Geometry: final body of the model. Coordinates: model frame, mm. Face numbers are marked on the shaded views. A direction names the side the tool comes from. Give positions to 0.01 mm unless a question says otherwise; leave off trailing zeros. Loops run counter-clockwise (first coordinate to the right, second up) from the corner with the lowest first, then second, coordinate; pieces in that order, holes last.
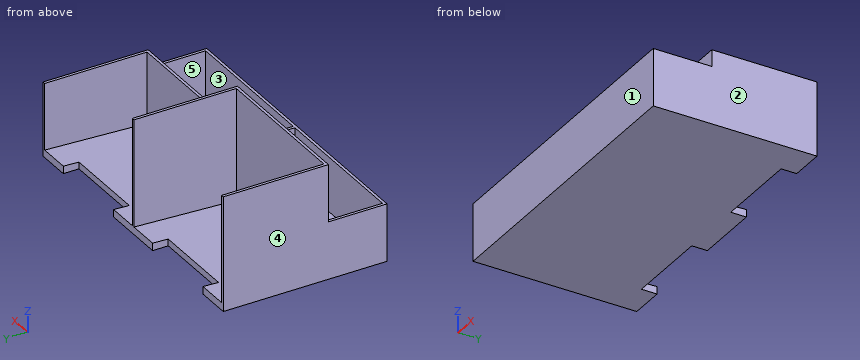
```python
from build123d import *

# Parameters (mm, degrees)
SKETCH1_W               = 193.4
SKETCH1_H               = 104.8
BOSS_EXTRUDE1_DEPTH     = 1.8
SKETCH1_8_W             = 1.8
SKETCH1_8_H             = 65.5
SKETCH1_8_H_2           = 1.8
SKETCH1_8_W_2           = 94
BOSS_EXTRUDE2_DEPTH     = 71.7
SKETCH1_10_W            = 94
SKETCH1_10_H            = 1.8
SKETCH1_10_W_2          = 1.8
SKETCH1_10_H_2          = 65.5
BOSS_EXTRUDE3_DEPTH     = 45.7
BOSS_EXTRUDE4_DEPTH     = 35
BOSS_EXTRUDE8_REACH     = 231.858
CUT_EXTRUDE1_DEPTH      = 27
CUT_EXTRUDE1_DEPTH_BACK = 16
SKETCH1_12_W            = 54
SKETCH1_12_H            = 10


with BuildPart() as part:
    # Sketch1 → Boss-Extrude1 (new body)
    with BuildSketch(Plane.XY):
        with Locations((96.7, 52.4)):
            Rectangle(SKETCH1_W, SKETCH1_H)
    extrude(amount=-BOSS_EXTRUDE1_DEPTH)

    # Sketch1<8> → Boss-Extrude2 (add)
    with BuildSketch(Plane.XY):
        with Locations((96.7, 72.05)):
            Rectangle(SKETCH1_8_W, SKETCH1_8_H)
        with Locations((96.7, 38.4)):
            Rectangle(SKETCH1_8_W, SKETCH1_8_H_2)
        with Locations((48.8, 38.4)):
            Rectangle(SKETCH1_8_W_2, SKETCH1_8_H_2)
        with Locations((0.9, 72.05)):
            Rectangle(SKETCH1_8_W, SKETCH1_8_H)
        with Locations((0.9, 38.4)):
            Rectangle(SKETCH1_8_W, SKETCH1_8_H_2)
    extrude(amount=BOSS_EXTRUDE2_DEPTH)

    # Sketch1<10> → Boss-Extrude3 (add)
    with BuildSketch(Plane.XY):
        with Locations((144.6, 38.4)):
            Rectangle(SKETCH1_10_W, SKETCH1_10_H)
        with Locations((192.5, 72.05)):
            Rectangle(SKETCH1_10_W_2, SKETCH1_10_H_2)
        with Locations((192.5, 38.4)):
            Rectangle(SKETCH1_10_W_2, SKETCH1_10_H)
    extrude(amount=BOSS_EXTRUDE3_DEPTH)

    # Sketch1<11> → Boss-Extrude4 (add)
    with BuildSketch(Plane.XY):
        Polygon((0, 37.5), (0, 0), (193.4, 0), (193.4, 37.5), (191.6, 37.5), (191.6, 1.8), (97.6, 1.8), (97.6, 37.5), (95.8, 37.5), (95.8, 1.8), (1.8, 1.8), (1.8, 37.5), align=None)
    extrude(amount=BOSS_EXTRUDE4_DEPTH)

    # Boss-Extrude8: up to this face of the body (flat: up to its plane)
    boss_extrude8_end = Plane(part.part.faces().sort_by_distance((1.8, 72.05, 35.85))[0])
    # Sketch2 → Boss-Extrude8 (add, up to the picked face)
    with BuildSketch(Plane.ZY.offset(-191.6), mode=Mode.PRIVATE) as boss_extrude8_sk1:
        Polygon((3, 104.8), (0, 104.8), (0, 39.3), align=None)
    boss_extrude8_tool1 = split(extrude(boss_extrude8_sk1.sketch, amount=BOSS_EXTRUDE8_REACH, mode=Mode.PRIVATE), bisect_by=boss_extrude8_end, keep=Keep.BOTH, mode=Mode.PRIVATE)
    add(boss_extrude8_tool1.solids().sort_by(Axis((191.6, 82.966667, 1), (-1, 0, 0)))[0])

    # Sketch1<12> → Cut-Extrude1 (cut, two sides: drawn at the far end of the back side and taken through both)
    with BuildSketch(Plane.XY.offset(-CUT_EXTRUDE1_DEPTH_BACK)):
        with Locations((144.6, 99.8)):
            Rectangle(SKETCH1_12_W, SKETCH1_12_H)
        with Locations((48.8, 99.8)):
            Rectangle(SKETCH1_12_W, SKETCH1_12_H)
    extrude(amount=CUT_EXTRUDE1_DEPTH + CUT_EXTRUDE1_DEPTH_BACK, mode=Mode.SUBTRACT)


solid = part.part
```
Q1. Mould query, pull axis Y, two halves, no side actions, for the marked faces 1, 2 and 3. Classes: +Y half, -Y half, draft (parallel to the pull), parting line (faces both ways), or undercut.
Q2. Section query D-D, the plane y = 51. Return loops of the section in (x, z).
Q3. Reachability of the marked faces 4 and 5 from +Z, -Z, +X, -X, +Y, -Y: full face, straight path, thin tool, end or side. Return the list, or none.
Q4. Material intervals for probe 1 along X at (y, z) = (17, 32.5); probe 2 along X at (y, z) = (54, 65); probe 3 along Y at (x, z) = (120.5, 23), sorted ascending.
Q5. Section query B-B, the plane x = 29.5. Return loops of the section in (y, z).
Q6. Section query C-C, the plane z = 61.5. Return loops of the section in (x, y), and give its area (3 significant figures).
Q7. Section query A-A, the plane z = 17. Return loops of the section in (x, y).
Q8. Pin query (flat end, axial travel): pin 1 Ø1.4 at (y, z) = (101.5, 0.5) entering from -X; pin 2 Ø2 at (x, z) = (90, 58.5) entering from +Y; pin 3 Ø5 at (x, z) = (146, 0.5) entering from +Y. Return the tip coordinate at first contact, or that it passes through.
Resolved:
1. face 1: -Y half
1. face 2: draft
1. face 3: undercut
2. outline: (0, -1.8) - (193.4, -1.8) - (193.4, 45.7) - (191.6, 45.7) - (191.6, 0.54) - (97.6, 0.54) - (97.6, 71.7) - (95.8, 71.7) - (95.8, 0.54) - (1.8, 0.54) - (1.8, 71.7) - (0, 71.7) - close
3. face 4: +Z, -Z, -X, +Y, -Y
3. face 5: +Z
4. probe 1: x = 0 to 1.8, 95.8 to 97.6, 191.6 to 193.4
4. probe 2: x = 0 to 1.8, 95.8 to 97.6
4. probe 3: y = 0 to 1.8, 37.5 to 39.3
5. outline: (0, -1.8) - (94.8, -1.8) - (94.8, 2.54) - (39.3, 0) - (39.3, 71.7) - (37.5, 71.7) - (37.5, 0) - (1.8, 0) - (1.8, 35) - (0, 35) - close
6. outline: (0, 37.5) - (97.6, 37.5) - (97.6, 104.8) - (95.8, 104.8) - (95.8, 39.3) - (1.8, 39.3) - (1.8, 104.8) - (0, 104.8) - close
6. area: 411 mm2
7. outline: (0, 0) - (193.4, 0) - (193.4, 104.8) - (191.6, 104.8) - (191.6, 39.3) - (97.6, 39.3) - (97.6, 104.8) - (95.8, 104.8) - (95.8, 39.3) - (1.8, 39.3) - (1.8, 104.8) - (0, 104.8) - close; hole (1.8, 1.8) - (95.8, 1.8) - (95.8, 37.5) - (1.8, 37.5) - close; hole (97.6, 1.8) - (191.6, 1.8) - (191.6, 37.5) - (97.6, 37.5) - close
8. pin 1: stops at x = 0
8. pin 2: stops at y = 39.3
8. pin 3: stops at y = 94.8
